Part model, mm, in its own coordinate system. Round coordinates to 2 decimals unless told otherwise and drop trailing zeros. Loops run counter-clockwise (first coordinate to the right, second up) from the corner with the lowest first, then second, coordinate; pieces in that order, holes last.
(1) Cut at C-C on y = 1.4. Count the separate pieces of the cut face and the enclosed holes in it, then the cut area to 3 significant figures.
(2) Cut at B-B on x = 90. List the corners of the cut face in (y, z) (3 decimals), then the cut area to 3 significant figures.
(3) Probe probe 1 along Z at (x, y) = (-115, 2.5); probe 2 along X at (y, z) = (0.95, 31.5). List the from-to ranges inside material, lowest first.
(4) Cut at A-A on z = 55. List the corners of the cut face in (x, y) (3 decimals).
(5) Flat gauge pins, fed straight in: pin 1 (8 mm diameter, centred on x = -105.5, z = -36, fed in from -Y); pin 2 (1.6 mm diameter, centred on y = 1, z = 36.5, fed in from -X); pin 3 (1 mm diameter, centred on x = -89, y = 1, fed in from +Z); pin 4 (1 mm diameter, centred on y = 1.5, z = 34.5, fed in from +X). Where does each tip first touch, or does it go through?
from build123d import *

# Parameters (mm, degrees)
SKETCH2_W           = 250
SKETCH2_H           = 250
BOSS_EXTRUDE1_DEPTH = 3.175
SKETCH3_W           = 8.6
SKETCH3_H           = 15.35
CUT_EXTRUDE1_DEPTH  = 10
SKETCH10_W          = 45
SKETCH10_H          = 3.175
BOSS_EXTRUDE2_DEPTH = 12.5
SKETCH11_W          = 45
SKETCH11_H          = 3.175
BOSS_EXTRUDE3_DEPTH = 12.5
SKETCH13_W          = 45
SKETCH13_H          = 3.175
BOSS_EXTRUDE4_DEPTH = 12.5
SKETCH14_W          = 45
SKETCH14_H          = 3.175
BOSS_EXTRUDE5_DEPTH = 12.5
M3_TAPPED_HOLE1_D   = 2.5
SKETCH21_R          = 1.25
CUT_EXTRUDE2_DEPTH  = 10
SKETCH22_R          = 1.651881978
SKETCH22_R_2        = 1.65156012
SKETCH22_R_3        = 1.651864629
SKETCH22_R_4        = 1.651
CUT_EXTRUDE3_DEPTH  = 4.175


with BuildPart() as part:
    # Sketch2 → Boss-Extrude1 (new body)
    with BuildSketch(Plane(origin=(0, 0, 0), x_dir=(1, 0, 0), z_dir=(0, 1, 0))):
        Rectangle(SKETCH2_W, SKETCH2_H)
    extrude(amount=BOSS_EXTRUDE1_DEPTH)

    # Sketch3 → Cut-Extrude1 (cut)
    with BuildSketch(Plane(origin=(0, 3.175, 0), x_dir=(1, 0, 0), z_dir=(0, 1, 0))):
        with Locations((-43.75, 35.675)):
            Rectangle(SKETCH3_W, SKETCH3_H)
        with Locations((-43.75, -35.675)):
            Rectangle(SKETCH3_W, SKETCH3_H)
        with Locations((43.75, -35.675)):
            Rectangle(SKETCH3_W, SKETCH3_H)
        with Locations((43.75, 35.675)):
            Rectangle(SKETCH3_W, SKETCH3_H)
    extrude(amount=-CUT_EXTRUDE1_DEPTH, mode=Mode.SUBTRACT)

    # Sketch10 → Boss-Extrude2 (add)
    with BuildSketch(Plane(origin=(0, 0, -125), x_dir=(-1, 0, 0), z_dir=(0, 0, -1))):
        with Locations((0, 1.5875)):
            Rectangle(SKETCH10_W, SKETCH10_H)
    extrude(amount=BOSS_EXTRUDE2_DEPTH)

    # Sketch11 → Boss-Extrude3 (add)
    with BuildSketch(Plane.ZY.offset(125)):
        with Locations((0, 1.5875)):
            Rectangle(SKETCH11_W, SKETCH11_H)
    extrude(amount=BOSS_EXTRUDE3_DEPTH)

    # Sketch13 → Boss-Extrude4 (add)
    with BuildSketch(Plane.XY.offset(125)):
        with Locations((0, 1.5875)):
            Rectangle(SKETCH13_W, SKETCH13_H)
    extrude(amount=BOSS_EXTRUDE4_DEPTH)

    # Sketch14 → Boss-Extrude5 (add)
    with BuildSketch(Plane(origin=(125, 0, 0), x_dir=(0, 0, -1), z_dir=(1, 0, 0))):
        with Locations((0, 1.5875)):
            Rectangle(SKETCH14_W, SKETCH14_H)
    extrude(amount=BOSS_EXTRUDE5_DEPTH)

    # M3 Tapped Hole1 (through all)
    with Locations(Plane(origin=(-115, 3.175, -115), x_dir=(0, 0, 1), z_dir=(0, 1, 0))):
        with Locations((0, 0)):
            Hole(M3_TAPPED_HOLE1_D / 2)

    # Sketch21 → Cut-Extrude2 (cut)
    with BuildSketch(Plane(origin=(0, 3.175, 0), x_dir=(1, 0, 0), z_dir=(0, 1, 0))):
        with Locations((115, 115)):
            Circle(SKETCH21_R)
        with Locations((115, -115)):
            Circle(SKETCH21_R)
        with Locations((-115, -115)):
            Circle(SKETCH21_R)
    extrude(amount=-CUT_EXTRUDE2_DEPTH, mode=Mode.SUBTRACT)

    # Sketch22 → Cut-Extrude3 (cut, through all)
    with BuildSketch(Plane(origin=(0, 3.175, 0), x_dir=(1, 0, 0), z_dir=(0, 1, 0))):
        with Locations((-89.96501808, -68.404219496)):
            Circle(SKETCH22_R)
        with Locations((-69.644539433, -68.404527337)):
            Circle(SKETCH22_R_2)
        with Locations((-69.644998895, -88.724239252)):
            Circle(SKETCH22_R_3)
        with Locations((-89.965017771, -88.724219998)):
            Circle(SKETCH22_R_4)
    extrude(amount=-CUT_EXTRUDE3_DEPTH, mode=Mode.SUBTRACT)


solid = part.part
Final values:
1. separate pieces: 1
1. enclosed holes: 12
1. area: 64,200 mm2
2. outline: (0, -125) - (3.175, -125) - (3.175, 125) - (0, 125) - close
2. area: 794 mm2
3. probe 1: z = -125 to -116.25, -113.75 to 113.75, 116.25 to 125
3. probe 2: x = -125 to -48.05, -39.45 to 39.45, 48.05 to 125
4. outline: (-125, 0) - (125, 0) - (125, 3.175) - (-125, 3.175) - close
5. pin 1: stops at y = 0
5. pin 2: stops at x = -125
5. pin 3: stops at z = 125
5. pin 4: stops at x = 125
